from build123d import *

# Parameters (mm, degrees)
SKETCH1_W           = 200
SKETCH1_H           = 200
BOSS_EXTRUDE1_DEPTH = 250
SKETCH2_W           = 220
SKETCH2_H           = 220
BOSS_EXTRUDE3_DEPTH = 5
SKETCH3_W           = 220
SKETCH3_H           = 220
BOSS_EXTRUDE4_DEPTH = 5
SKETCH4_W           = 190
SKETCH4_H           = 190
CUT_EXTRUDE1_DEPTH  = 251


with BuildPart() as part:
    # Sketch1 → Boss-Extrude1 (new body)
    with BuildSketch(Plane.XY):
        Rectangle(SKETCH1_W, SKETCH1_H)
    extrude(amount=BOSS_EXTRUDE1_DEPTH)

    # Sketch2 → Boss-Extrude3 (add)
    with BuildSketch(Plane.XY.offset(250)):
        Rectangle(SKETCH2_W, SKETCH2_H)
    extrude(amount=-BOSS_EXTRUDE3_DEPTH)

    # Sketch3 → Boss-Extrude4 (add)
    with BuildSketch(Plane(origin=(0, 0, 0), x_dir=(-1, 0, 0), z_dir=(0, 0, -1))):
        Rectangle(SKETCH3_W, SKETCH3_H)
    extrude(amount=-BOSS_EXTRUDE4_DEPTH)

    # Sketch4 → Cut-Extrude1 (cut, through all)
    with BuildSketch(Plane.XY.offset(250)):
        Rectangle(SKETCH4_W, SKETCH4_H)
    extrude(amount=-CUT_EXTRUDE1_DEPTH, mode=Mode.SUBTRACT)


solid = part.part
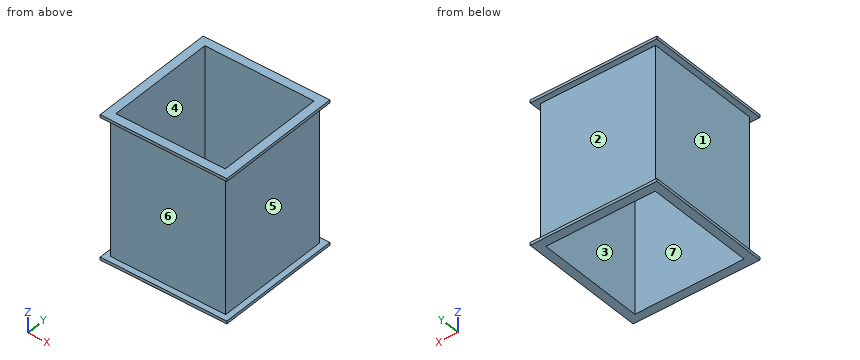
Design review of the part built by this model. Coordinates are the model's own, in mm. Face numbers are marked on the shaded views. A direction names the side the tool comes from. Give positions to 0.01 mm unless a question says otherwise; leave off trailing zeros. Loops run counter-clockwise (first coordinate to the right, second up) from the corner with the lowest first, then second, coordinate; pieces in that order, holes last. Notation, with made-up numbers: (70.25, 42) - (108.25, 42) arc R19 cw to (108.25, 64) - close; hole circle Ø4 at (-32, 71.5). An arc over 180 degrees is marked (long way). Use CSV: the item, a comma, the result in double quotes. Start each with the question number.
1. Insertion check: P1, Ø6, axis at x = 45.5, z = 192, coming from the +Y side; P2, Ø1.5, axis at y = -19.5, z = 105, coming from the -X side; P3, Ø1, axis at y = 32.5, z = 103, coming from the +X side. Each pin has a flat end and moves straight along its axis. Give the tip position at first contact, or say it passes through.
2. Add section C-C (z = 78.5). State the section outline as (x, y) points, plus the area to 3 significant figures.
3. Wall thickness on L1, parallel to X at y = -4, z = 67.5; L2, parallel to X at y = 99.5, z = 231: over which ranges is each line inside the solid? List them lowest first.
4. Draft analysis for pull direction Y (two halves, no side actions). For the marked faces 1, 2, 3 and 4, state which applies: released by +Y, released by -Y, zero draft, split by the parting line, or undercut.
5. Add section A-A (x = 54.5). State the section outline as (y, z) points, plus the area to 3 significant figures.
6. Machinability: for the marked faces 5, 6 and 7, which of the approach directions +Z, -Z, +X, -X, +Y, -Y give a long, thin tool a straight path to every point of the face, cutting with its end or side? Answer none if there is none.
Results found:
1,P1,"stops at y = 100"
1,P2,"stops at x = -100"
1,P3,"stops at x = 100"
2,outline,"(-100, -100) - (100, -100) - (100, 100) - (-100, 100) - close; hole (-95, -95) - (95, -95) - (95, 95) - (-95, 95) - close"
2,area,"3,900 mm²"
3,L1,"x = -100 to -95, 95 to 100"
3,L2,"x = -100 to 100"
4,face 1,"zero draft"
4,face 2,"released by +Y"
4,face 3,"undercut"
4,face 4,"undercut"
5,outline,"(-110, 0) - (-95, 0) - (-95, 250) - (-110, 250) - (-110, 245) - (-100, 245) - (-100, 5) - (-110, 5) - close; (95, 0) - (110, 0) - (110, 5) - (100, 5) - (100, 245) - (110, 245) - (110, 250) - (95, 250) - close"
5,area,"2,700 mm²"
6,face 5,"+X, +Y, -Y"
6,face 6,"+X, -X, -Y"
6,face 7,"+Z, -Z"
